Input: dimensioned drawing with shaded views. Units: mm. Origin: part minimum x, y, z. A direction names the side the tool comes from. Round coordinates to 2 decimals unless told otherwise and drop trailing zeros. Loops run counter-clockwise (first coordinate to the right, second up) from the corner with the lowest first, then second, coordinate; pieces in that order, holes last. Notation, with made-up numbers: M -5,27 L 46,27 A19 ccw 46,56 Z; hole C 47.5,76.5 d9. An arc over 180 degrees is marked long. Put each result on its own line as item: value. Start each with the question number.
1) Reachability of the marked faces 1 and 2 from +Z, -Z, +X, -X, +Y, -Y: full face, straight path, thin tool, end or side. Return the list, or none.
2) Section C-C on z = 4. Output: boundary loops of the cut face in (x, y), plus the area to 3 significant figures.
3) Pin query (flat end, axial travel): pin 1 (14.5 mm diameter, centred on x = 18, y = 9, fed in from -Z); pin 2 (3 mm diameter, centred on y = 4, z = 6.5, fed in from +X); pin 3 (4 mm diameter, centred on y = 22.5, z = 3, fed in from +X); pin 4 (3 mm diameter, centred on y = 11.5, z = 1.5, fed in from -X). Return the tip coordinate at first contact, or that it passes through.
4) Section A-A on y = 14.5. Output: boundary loops of the cut face in (x, z).
5) Line query: probe 1 along Z at (x, y) = (24.75, 20.25); probe 2 along Y at (x, z) = (25, 7); probe 3 along X at (y, z) = (14, 1.75). Output: solid intervals per line, ascending.
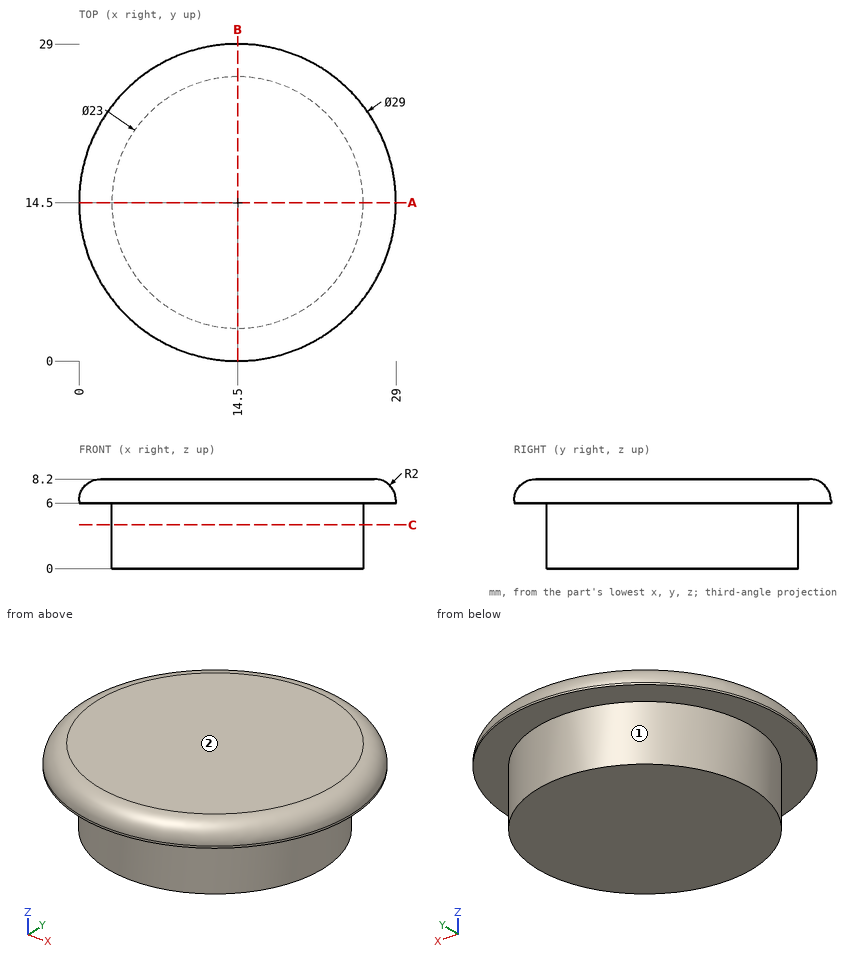
Geometry results:
1. face 1: -Z
1. face 2: +Z, +X, -X, +Y, -Y
2. outline: C 14.5,14.5 d23
2. area: 415 mm²
3. pin 1: stops at z = 0
3. pin 2: stops at x = 25.86
3. pin 3: stops at x = 24.31
3. pin 4: stops at x = 3.1
4. outline: M 0,6 L 3,6 L 3,0 L 26,0 L 26,6 L 29,6 L 29,6.2 A2 ccw 27,8.2 L 2,8.2 A2 ccw 0,6.2 Z
5. probe 1: z = 6 to 8.2
5. probe 2: y = 4.74 to 24.26
5. probe 3: x = 3.01 to 25.99
